Source: CAD feature listing. Evaluate the final solid. Frame: model axes, mm. A direction names the side the tool comes from. Coordinates: 2 decimals unless noted, no trailing zeros. Write each loop counter-clockwise with the first axis right and the second up, starting at its lowest first coordinate (ties: lowest second). Pieces come first, ordered by that corner, then holes. Notation, with made-up numbers: (43, 53) - (95, 53) arc R25 ccw to (95, 86) - close; hole circle Ø1 at (-6, 19.5). An arc over 180 degrees is marked (long way). One line per question, with ' | ' between items.
from build123d import *

# Parameters (mm, degrees)
SKETCH1_R           = 1
BOSS_EXTRUDE1_DEPTH = 2


with BuildPart() as part:
    # Sketch1 → Boss-Extrude1 (new body)
    with BuildSketch(Plane.XY):
        with BuildLine():
            Line((0, -2), (0, 2))
            Line((0, 2), (12, 2))
            ThreePointArc((12, 2), (12.632455532, 2.102633404), (13.2, 2.4))
            ThreePointArc((13.2, 2.4), (18, 0), (13.2, -2.4))
            ThreePointArc((13.2, -2.4), (12.632455532, -2.102633404), (12, -2))
            Line((12, -2), (0, -2))
        make_face()
        with Locations((15, 0)):
            Circle(SKETCH1_R, mode=Mode.SUBTRACT)
    boss_extrude1 = extrude(amount=BOSS_EXTRUDE1_DEPTH)

    # Mirror1: Boss-Extrude1 across plane
    add(boss_extrude1.mirror(Plane(origin=(0, -2, 2), x_dir=(0, 0, 1), z_dir=(-1, 0, 0))))


solid = part.part
Item 1: Cut plane C-C on z = 1.5. Return loops of the section in (x, y).
Check sheet entries:
outline: (-13.2, -2.4) arc R2 cw to (-12, -2) - (12, -2) arc R2 cw to (13.2, -2.4) arc R3 ccw (long way) to (13.2, 2.4) arc R2 cw to (12, 2) - (-12, 2) arc R2 cw to (-13.2, 2.4) arc R3 ccw (long way) to start; hole circle Ø2 at (-15, 0); hole circle Ø2 at (15, 0)
Item 2: Cut plane B-B on y = 0. Return loops of the section in (x, z), and give its area (3 significant figures).
Check sheet entries:
outline: (-18, 0) - (-16, 0) - (-16, 2) - (-18, 2) - close; (-14, 0) - (14, 0) - (14, 2) - (-14, 2) - close; (16, 0) - (18, 0) - (18, 2) - (16, 2) - close | area: 64.0 mm²
Item 3: Cut plane D-D on x = -11.5. Return loops of the section in (y, z).
Check sheet entries:
outline: (-2, 0) - (2, 0) - (2, 2) - (-2, 2) - close
Item 4: Cut plane A-A on x = 15. Return loops of the section in (y, z), and give its area (3 significant figures).
Check sheet entries:
outline: (-3, 0) - (-1, 0) - (-1, 2) - (-3, 2) - close; (1, 0) - (3, 0) - (3, 2) - (1, 2) - close | area: 8.00 mm²
Item 5: Mould query, pull axis X, two halves, no side actions, for faces 1 (the face through (-16, 0, 1)), 2 (the face through (0, 0, 0)). Classes: pulls with the +X half, pulls with the -X half, needs draft (parallel to the pull), parting line crosses it, or undercut.
Check sheet entries:
face 1: undercut | face 2: needs draft
Item 6: Pin query (flat end, axial travel): pin 1 Ø0.6 at (x, z) = (-4.5, 0.5) entering from -Y. Return the tip coordinate at first contact, or that it passes through.
Check sheet entries:
pin 1: y = -2
Item 7: Ray query, line 1 along Y through (x, z) = (15, 0.95); line 2 along X through (y, z) = (0.55, 0.7); line 3 along Y through (x, z) = (-0.5, 0.75). Return the intervals inside material, ascending. Write a range as [from, to].
Check sheet entries:
line 1: [-3, -1], [1, 3] | line 2: [-17.95, -15.84], [-14.16, 14.16], [15.84, 17.95] | line 3: [-2, 2]
Item 8: Access query for faces 3 (the face through (0, 0, 2)), 4 (the face through (12.641, -2.106, 0.986)), 5 (the face through (12.62, 2.1, 0.99)). Directions: +Z, -Z, +X, -X, +Y, -Y. A direction counts if a zero-diameter tool reaches every point of the face in a straight line with its end or side. Return the directions, or none.
Check sheet entries:
face 3: +Z, +X, -X, +Y, -Y | face 4: +Z, -Z, -Y | face 5: +Z, -Z, +Y
